Verification items for the finished model (mm, model axes). A direction names the side the tool comes from. Coordinates: 2 decimals unless noted, no trailing zeros. Write each loop counter-clockwise with the first axis right and the second up, starting at its lowest first coordinate (ties: lowest second). Pieces come first, ordered by that corner, then holes. Notation, with made-up numbers: (14.5, -25) -> (34.5, -25) arc R25 cw to (34.5, -12) -> close; hole circle Ø11 at (89.25, 55). An arc over 180 degrees is marked (long way). Answer in a Markdown table with one row per item.
```python
from build123d import *

# Parameters (mm, degrees)
F0_W     = 130
F0_H     = 93
F3_DEPTH = 5
F1_W     = 126
F1_H     = 89
F4_DEPTH = 1.8
F2_W     = 108.2
F2_H     = 65
F5_DEPTH = 25
F6_SIZE  = 2.5


with BuildPart() as f3:
    # F0 (on Front) → F3 (new body)
    with BuildSketch(Plane.XZ):
        with Locations((-5.6, -8.7)):
            Rectangle(F0_W, F0_H)
    extrude(amount=F3_DEPTH)

    # F1 (on face) → F4 (cut)
    with BuildSketch(Plane.XZ):
        with Locations((-5.6, -8.7)):
            Rectangle(F1_W, F1_H)
    extrude(amount=F4_DEPTH, mode=Mode.SUBTRACT)

    # F2 (on face) → F5 (cut)
    with BuildSketch(Plane.XZ):
        with Locations((-5.6, -6.7)):
            Rectangle(F2_W, F2_H)
    extrude(amount=F5_DEPTH, mode=Mode.SUBTRACT)

    # F6
    f6_edges = [f3.edges().sort_by_distance(p)[0] for p in [
        (-5.6, -5, 25.8),
        (-59.7, -5, -6.7),
        (48.5, -5, -6.7),
        (-5.6, -5, -39.2),
        (-70.6, -5, -8.7),
        (-5.6, -5, -55.2),
        (-5.6, -5, 37.8),
        (59.4, -5, -8.7),
    ]]
    chamfer(f6_edges, length=F6_SIZE)


solid = f3.part
```
1. Section check B-B, the plane z = 3.5. Record the boundary of the cut face in (x, y), plus the area to 3 significant figures.
Geometry says:
| item | result |
|---|---|
| outline | (-70.6, -2.5) -> (-68.1, -5) -> (-62.2, -5) -> (-59.7, -2.5) -> (-59.7, -1.8) -> (-68.6, -1.8) -> (-68.6, 0) -> (-70.6, 0) -> close; (48.5, -2.5) -> (51, -5) -> (56.9, -5) -> (59.4, -2.5) -> (59.4, 0) -> (57.4, 0) -> (57.4, -1.8) -> (48.5, -1.8) -> close |
| area | 64.5 mm^2 |
2. Depth check by flat-ended pin: P1, Ø1.5, axis at y = -4.5, z = 12.5, coming from the -X side. Enter the tip coordinate at first touch or a pass-through.
Geometry says:
| item | result |
|---|---|
| P1 | x = -69.35 |
3. Mould release check, pull along Z, two halves, no side actions. Record for faces 1 (the flat face through (-6, -1.8, -48)), 2 (the flat face through (-69.3, -3.8, -9.4)), 3 (the flat face through (-6.5, -3.8, 36.5)): released by +Z, released by -Z, zero draft, split by the parting line, or undercut.
Geometry says:
| item | result |
|---|---|
| face 1 | undercut |
| face 2 | zero draft |
| face 3 | released by +Z |
4. Section check D-D, the plane z = -43.5. Record the boundary of the cut face in (x, y), plus the area to 3 significant figures.
Geometry says:
| item | result |
|---|---|
| outline | (-70.6, -2.5) -> (-68.1, -5) -> (56.9, -5) -> (59.4, -2.5) -> (59.4, 0) -> (57.4, 0) -> (57.4, -1.8) -> (-68.6, -1.8) -> (-68.6, 0) -> (-70.6, 0) -> close |
| area | 417 mm^2 |
5. Section check A-A, the plane x = 1. Record the boundary of the cut face in (y, z), plus the area to 3 significant figures.
Geometry says:
| item | result |
|---|---|
| outline | (-5, -52.7) -> (-2.5, -55.2) -> (0, -55.2) -> (0, -53.2) -> (-1.8, -53.2) -> (-1.8, -39.2) -> (-2.5, -39.2) -> (-5, -41.7) -> close; (-5, 28.3) -> (-2.5, 25.8) -> (-1.8, 25.8) -> (-1.8, 35.8) -> (0, 35.8) -> (0, 37.8) -> (-2.5, 37.8) -> (-5, 35.3) -> close |
| area | 84.3 mm^2 |
6. Tool access check on faces 4 (the flat face through (-6.5, -3.8, -53.9)), 5 (the flat face through (-4.8, -3.7, 27)). Record the directions out of +Z, -Z, +X, -X, +Y, -Y that give a thin tool (end or side, any length) a straight path to the whole face; none if there is none.
Geometry says:
| item | result |
|---|---|
| face 4 | -Z, +X, -X, -Y |
| face 5 | -Y |
7. Thickness scan on line 1 (X direction, y = -2.25, z = 14); line 2 (X direction, y = -1.05, z = -25); line 3 (Z direction, x = 3, y = -1.45). Record the ranges inside material, lowest first. Write a range as from..to.
Geometry says:
| item | result |
|---|---|
| line 1 | -70.6..-59.7, 48.5..59.4 |
| line 2 | -70.6..-68.6, 57.4..59.4 |
| line 3 | -55.2..-53.2, 35.8..37.8 |
8. Section check C-C, the plane y = -4.2. Record the boundary of the cut face in (x, z), plus the area to 3 significant figures.
Geometry says:
| item | result |
|---|---|
| outline | (-68.9, -53.5) -> (57.7, -53.5) -> (57.7, 36.1) -> (-68.9, 36.1) -> close; hole (-61.4, -40.9) -> (50.2, -40.9) -> (50.2, 27.5) -> (-61.4, 27.5) -> close |
| area | 3,710 mm^2 |
